```python
from build123d import *

# Parameters (mm, degrees)
SKETCH_9_R           = 40.020028018
SKETCH_9_R_2         = 2
EXTRUDE_3_DEPTH      = 7
EXTRUDE_4_DEPTH      = 7
EXTRUDE_4_DEPTH_BACK = 4
CUT_EXTRUDE_4_DEPTH  = 4
SKETCH_12_RX         = 39
SKETCH_12_RY         = 4.15
CUT_EXTRUDE_6_DEPTH  = 2
SKETCH_13_R          = 4.15
CUT_EXTRUDE_7_DEPTH  = 57.914016597


with BuildPart() as part:
    # Sketch 9 → Extrude 3 (new body)
    with BuildSketch(Plane(origin=(0, 0, 0), x_dir=(1, 0, 0), z_dir=(0, 1, 0))):
        with Locations(Location((0, 0, 0), (0, 0, 270))):
            Circle(SKETCH_9_R)
        with Locations(Location((-28.746176582, -21.437246172, 0), (0, 0, 270))):
            Circle(SKETCH_9_R_2, mode=Mode.SUBTRACT)
        with Locations(Location((-12.481803809, -34.453899709, 0), (0, 0, 270))):
            Circle(SKETCH_9_R_2, mode=Mode.SUBTRACT)
        with Locations(Location((12.482594231, -34.454465093, 0), (0, 0, 270))):
            Circle(SKETCH_9_R_2, mode=Mode.SUBTRACT)
        with Locations(Location((28.804113616, -21.353828271, 0), (0, 0, 270))):
            Circle(SKETCH_9_R_2, mode=Mode.SUBTRACT)
    extrude(amount=EXTRUDE_3_DEPTH)

    # Sketch 9_3 → Extrude 4 (add, two sides: drawn at the far end of the back side and taken through both)
    with BuildSketch(Plane(origin=(0, 0, 0), x_dir=(1, 0, 0), z_dir=(0, 1, 0)).offset(-EXTRUDE_4_DEPTH_BACK)):
        with BuildLine():
            ThreePointArc((-26.746176582, -21.437246172), (-27.778871949, -19.686725751), (-29.810498329, -19.743959658))
            ThreePointArc((-29.810498329, -19.743959658), (-28.746176582, -21.437246172), (-27.585789036, -23.066203122))
            ThreePointArc((-27.585789036, -23.066203122), (-26.968428696, -22.353549864), (-26.746176582, -21.437246172))
        make_face()
        with BuildLine():
            ThreePointArc((-27.585789036, -23.066203122), (-28.746176582, -21.437246172), (-29.810498329, -19.743959658))
            ThreePointArc((-29.810498329, -19.743959658), (-30.407992627, -22.550065759), (-27.585789036, -23.066203122))
        make_face()
        with BuildLine():
            ThreePointArc((-10.481803809, -34.453899709), (-12.086387614, -32.493377831), (-14.325449842, -33.678677608))
            ThreePointArc((-14.325449842, -33.678677608), (-12.481803809, -34.453899709), (-10.596443163, -35.12129407))
            ThreePointArc((-10.596443163, -35.12129407), (-10.51067199, -34.792484046), (-10.481803809, -34.453899709))
        make_face()
        with BuildLine():
            ThreePointArc((-10.596443163, -35.12129407), (-12.481803809, -34.453899709), (-14.325449842, -33.678677608))
            ThreePointArc((-14.325449842, -33.678677608), (-13.203413531, -36.31918237), (-10.596443163, -35.12129407))
        make_face()
        with BuildLine():
            ThreePointArc((14.326275376, -33.679326501), (11.761068998, -32.589149748), (10.597203357, -35.121774056))
            ThreePointArc((10.597203357, -35.121774056), (12.482594231, -34.454465093), (14.326275376, -33.679326501))
        make_face()
        with BuildLine():
            ThreePointArc((14.326275376, -33.679326501), (12.482594231, -34.454465093), (10.597203357, -35.121774056))
            ThreePointArc((10.597203357, -35.121774056), (12.821133927, -36.425604579), (14.482594231, -34.454465093))
            ThreePointArc((14.482594231, -34.454465093), (14.443125064, -34.059093299), (14.326275376, -33.679326501))
        make_face()
        with BuildLine():
            ThreePointArc((29.863522136, -19.657463456), (27.139078544, -20.245830883), (27.648453212, -22.986142282))
            ThreePointArc((27.648453212, -22.986142282), (28.804113616, -21.353828271), (29.863522136, -19.657463456))
        make_face()
        with BuildLine():
            ThreePointArc((29.863522136, -19.657463456), (28.804113616, -21.353828271), (27.648453212, -22.986142282))
            ThreePointArc((27.648453212, -22.986142282), (29.722993149, -23.130246128), (30.804113616, -21.353828271))
            ThreePointArc((30.804113616, -21.353828271), (30.553230113, -20.383987315), (29.863522136, -19.657463456))
        make_face()
    extrude(amount=EXTRUDE_4_DEPTH + EXTRUDE_4_DEPTH_BACK)

    # Sketch 10 → Cut-Extrude 4 (cut)
    with BuildSketch(Plane(origin=(0, 7, 0), x_dir=(1, 0, 0), z_dir=(0, 1, 0))):
        Polygon((39, 0), (0, 0), (-39, 0), (-39, -4.15), (39, -4.15), align=None)
        Polygon((-39, 0), (0, 0), (39, 0), (39, 4.15), (-39, 4.15), align=None)
    extrude(amount=-CUT_EXTRUDE_4_DEPTH, mode=Mode.SUBTRACT)

    # Sketch 12 → Cut-Extrude 6 (cut)
    with BuildSketch(Plane(origin=(0, 3, 0), x_dir=(1, 0, 0), z_dir=(0, 1, 0))):
        with Locations(Location((0, 0), (0, 0, 0))):
            Ellipse(SKETCH_12_RX, SKETCH_12_RY)
    extrude(amount=-CUT_EXTRUDE_6_DEPTH, mode=Mode.SUBTRACT)

    # Sketch 13 → Cut-Extrude 7 (cut, through all)
    with BuildSketch(Plane(origin=(0, 1, 0), x_dir=(1, 0, 0), z_dir=(0, 1, 0))):
        with Locations(Location((0, 0, 0), (0, 0, 270))):
            Circle(SKETCH_13_R)
    extrude(amount=-CUT_EXTRUDE_7_DEPTH, mode=Mode.SUBTRACT)


solid = part.part
```
For this review, take the finished solid that the model builds, in its own axes (mm). A direction names the side the tool comes from. Coordinates: 2 decimals unless noted, no trailing zeros. Write each loop counter-clockwise with the first axis right and the second up, starting at its lowest first coordinate (ties: lowest second). Pieces come first, ordered by that corner, then holes.
(1) Add section C-C on z = -24. Give the boundary of the cut face in (x, y), then the cut area to 3 significant figures.
(2) The part is to be moulded in two halves that separate along Z. For faces 1 (the face through (1, 7, 8)), 2 (the face through (-39, 5, 0)), 3 (the face through (33.75, 3.45, 21.51)), say which applies: +Z half, -Z half, draft (parallel to the pull), parting line (faces both ways), or undercut.
(3) For pin 1 Ø4.5 at (x, z) = (17.5, 2.5) entering from +Y; pin 2 Ø3 at (y, z) = (4, 19.5) entering from +X; pin 3 Ø4.5 at (x, y) = (-7, 4.5) entering from -Z; pin 4 Ø5 at (x, z) = (0, 0) entering from +Y, all flat-tipped, find the tip position at first contact; note any pin that passes through.
(4) Wall thickness on probe 1 along Z at (x, y) = (0.5, 5.5); probe 2 along Y at (x, z) = (-20, 25): over which ranges is each line inside the solid? List them lowest first.
(5) Add section B-B on y = 5.75. Give the boundary of the cut face in (x, z), then the cut area to 3 significant figures.
(6) Add section D-D on z = 17. Give the boundary of the cut face in (x, y).
(7) Tool access review of faces 4 (the face through (-31, 3, 3)), 5 (the face through (-13, -4, 34)): name each direction out of +Z, -Z, +X, -X, +Y, -Y from which nothing blocks a thin tool from reaching the whole face with its end or side.
(8) Add section A-A on y = -2.25. Give the boundary of the cut face in (x, z).
Answer sheet:
1. outline: (-32.03, 0) - (32.03, 0) - (32.03, 7) - (-32.03, 7) - close
1. area: 448 mm2
2. face 1: draft
2. face 2: undercut
2. face 3: parting line
3. pin 1: stops at y = 7
3. pin 2: stops at x = 35.74
3. pin 3: stops at z = -39.74
3. pin 4: passes through
4. probe 1: z = -40.02 to -4.15, 4.15 to 40.02
4. probe 2: y = 0 to 7
5. outline: circle Ø80.04 at (0, 0); hole (-39, -4.15) - (39, -4.15) - (39, 4.15) - (-39, 4.15) - close
5. area: 4,380 mm2
6. outline: (-36.23, 0) - (36.23, 0) - (36.23, 7) - (-36.23, 7) - close
7. face 4: +Y
7. face 5: +Z, -Z, +X, -X, -Y
8. outline: circle Ø4 at (-28.75, 21.44); circle Ø4 at (-12.48, 34.45); circle Ø4 at (12.48, 34.45); circle Ø4 at (28.8, 21.35)
